```python
from build123d import *

# Parameters (mm, degrees)
EXTRUDE_1_DEPTH     = 3
SKETCH_2_R          = 1.6
CUT_EXTRUDE_1_DEPTH = 3
SKETCH_3_R          = 2.1
CUT_EXTRUDE_2_DEPTH = 3
CUT_EXTRUDE_3_DEPTH = 10
FILLET_1_R          = 10
FILLET_2_R          = 3


with BuildPart() as part:
    # 草图1 → 凸台-拉伸1 (new body)
    with BuildSketch(Plane(origin=(0, 0, 0), x_dir=(1, 0, 0), z_dir=(0, 1, 0))):
        with BuildLine():
            Line((-7.5, -30), (7.5, -30))
            Line((7.5, -30), (7.5, 30))
            ThreePointArc((7.5, 30), (0, 37.5), (-7.5, 30))
            Line((-7.5, 30), (-7.5, -30))
        make_face()
    extrude(amount=EXTRUDE_1_DEPTH)

    # 草图2 → 切除-拉伸1 (cut)
    with BuildSketch(Plane(origin=(0, 3, 0), x_dir=(1, 0, 0), z_dir=(0, 1, 0))):
        with Locations(Location((0, 30, 0), (0, 0, 270))):
            Circle(SKETCH_2_R)
    extrude(amount=-CUT_EXTRUDE_1_DEPTH, mode=Mode.SUBTRACT)

    # 草图3 → 切除-拉伸2 (cut)
    with BuildSketch(Plane.XZ):
        with Locations(Location((0, 20, 0), (0, 0, 270))):
            Circle(SKETCH_3_R)
        with Locations(Location((0, 0, 0), (0, 0, 270))):
            Circle(SKETCH_3_R)
    extrude(amount=-CUT_EXTRUDE_2_DEPTH, mode=Mode.SUBTRACT)

    # 草图4 → 切除-拉伸3 (cut)
    with BuildSketch(Plane.XZ):
        Polygon((-7.5, -12.5), (-4.9980923, -12.5), (-4.9980923, 27.5), (5.0019077, 27.5), (5.0019077, -12.5), (7.5, -12.5), (7.5, 30), (-7.5, 30), align=None)
    extrude(amount=-CUT_EXTRUDE_3_DEPTH, mode=Mode.SUBTRACT)

    # 圆角1
    # the kernel refuses this fillet: 10 mm, written as the material it takes off along each edge
    with BuildSketch(Plane(origin=(7.5, -16.5305363, -12.5), x_dir=(0, 0, -1), z_dir=(0, 1, 0))) as fillet_1_piece_1:
        with BuildLine():
            CenterArc((6.61221452, 10), FILLET_1_R, 228.606905679, 41.393094321)
            Line((0, 2.4980923), (-0.13224429, 2.348054146))
            ThreePointArc((-0.13224429, 2.348054146), (-0.2, 1.24904615), (-0.2, 0))
            Line((-0.2, 0), (0, -0.2))
            Line((0, -0.2), (6.61221452, -0.2))
            Line((6.61221452, -0.2), (6.61221452, 0))
        make_face()
    extrude(amount=36.061072601, mode=Mode.SUBTRACT)
    with BuildSketch(Plane(origin=(-7.5, -16.541351944, -12.5), x_dir=(0, 0, -1), z_dir=(0, 1, 0))) as fillet_1_piece_2:
        with BuildLine():
            CenterArc((6.616540778, -10), FILLET_1_R, 90, 41.426144493)
            Line((0, -2.5019077), (-0.132330816, -2.351945854))
            ThreePointArc((-0.132330816, -2.351945854), (-0.2, -1.25095385), (-0.2, 0))
            Line((-0.2, 0), (0, 0.2))
            Line((0, 0.2), (6.616540778, 0.2))
            Line((6.616540778, 0.2), (6.616540778, 0))
        make_face()
    extrude(amount=36.082703888, mode=Mode.SUBTRACT)

    # 圆角2
    fillet_2_edges = [part.edges().sort_by_distance(p)[0] for p in [
        (5.0019077, 1.5, 27.5),
        (-4.9980923, 1.5, 27.5),
    ]]
    fillet(fillet_2_edges, radius=FILLET_2_R)


solid = part.part
```
Check sheet for the modelled part. Datum: model origin and axes. Units: mm. A direction names the side the tool comes from. Coordinates: 2 decimals unless noted, no trailing zeros. Write each loop counter-clockwise with the first axis right and the second up, starting at its lowest first coordinate (ties: lowest second). Pieces come first, ordered by that corner, then holes. Notation, with made-up numbers: (-39, 37.5) -> (20, 37.5) arc R12 ccw to (20, 44.5) -> close; hole circle Ø8 at (-15.5, -38.5). An arc over 180 degrees is marked (long way). Use a Markdown table: item, result.
1. Sectioned sample at B-B (y = 1.05). Enter the section's corners in (x, z), plus the area to 3 significant figures.
Reported:
| item | result |
|---|---|
| outline | (-7.5, -30) arc R7.5 ccw to (7.5, -30) -> (7.5, -19.11) arc R10 ccw to (5, -12.5) -> (5, 24.5) arc R3 ccw to (2, 27.5) -> (-2, 27.5) arc R3 ccw to (-5, 24.5) -> (-5, -12.5) arc R10 ccw to (-7.5, -19.12) -> close; hole circle Ø4.2 at (0, 0); hole circle Ø4.2 at (0, 20); hole circle Ø3.2 at (0, -30) |
| area | 701 mm2 |
2. Sectioned sample at C-C (z = -11). Enter the section's corners in (x, y).
Reported:
| item | result |
|---|---|
| outline | (-5, 0) -> (5, 0) -> (5, 3) -> (-5, 3) -> close |
3. Sectioned sample at D-D (x = -6). Enter the section's corners in (y, z), plus the area to 3 significant figures.
Reported:
| item | result |
|---|---|
| outline | (0, -34.5) -> (3, -34.5) -> (3, -13.85) -> (0, -13.85) -> close |
| area | 62.0 mm2 |
4. Go/stop test with flat-tipped pins: pin 1 Ø1.5 at (y, z) = (1, 2.5) entering from +X; pin 2 Ø3.5 at (x, z) = (0, -30) entering from +Y; pin 3 Ø1 at (x, y) = (3, 1) entering from +Z. Record where each tip stops, or that it passes through.
Reported:
| item | result |
|---|---|
| pin 1 | stops at x = 5 |
| pin 2 | stops at y = 3 |
| pin 3 | stops at z = 27.46 |
5. Tool access check on faces 1 (the flat face through (5.002, 1, 6)), 2 (the flat face through (-4.998, 1, 6)), 3 (the cylindrical face through (0.16, 1.48, -37.5)). Record the directions out of +Z, -Z, +X, -X, +Y, -Y that give a thin tool (end or side, any length) a straight path to the whole face; none if there is none.
Reported:
| item | result |
|---|---|
| face 1 | +Z, +X, +Y, -Y |
| face 2 | +Z, -X, +Y, -Y |
| face 3 | -Z, +Y, -Y |
6. Scan lines: line 1 along X through (y, z) = (2.2, -30); line 2 along Z through (x, y) = (-1.25, 1.4); line 3 along X through (y, z) = (0.95, 20). Record each from-to range of solid material in increasing order.
Reported:
| item | result |
|---|---|
| line 1 | x = -7.5 to -1.6, 1.6 to 7.5 |
| line 2 | z = -37.4 to -31, -29 to -1.69, 1.69 to 18.31, 21.69 to 27.5 |
| line 3 | x = -5 to -2.1, 2.1 to 5 |
7. Sectioned sample at A-A (z = 20). Enter the section's corners in (x, y), plus the area to 3 significant figures.
Reported:
| item | result |
|---|---|
| outline | (-5, 0) -> (-2.1, 0) -> (-2.1, 3) -> (-5, 3) -> close; (2.1, 0) -> (5, 0) -> (5, 3) -> (2.1, 3) -> close |
| area | 17.4 mm2 |
